Autodesk Inventor part; units mm, degrees
ref_plane "YZ Plane" through (0, 0, 0) normal (1, 0, 0) x (0, 1, 0)
ref_plane "XZ Plane" through (0, 0, 0) normal (0, 1, 0) x (-1, 0, 0)
ref_plane "XY Plane" through (0, 0, 0) normal (0, 0, 1) x (1, 0, 0)
sketch "Boceto1" plane through (0, 0, 0) normal (0, 1, 0) x (-1, 0, 0)
  circle A0 centre (0, 0) radius 11
  arc A1 (-35, 0) -> (27, 22.2711) centre (0, 0) ccw
  line L0 (-35, 0) -> (-35, 75)
  line L1 (-35, 75) -> (27, 75)
  line L2 (27, 75) -> (27, 22.2711)
  arc A2 (-11, 45) -> (11, 45) centre (0, 45) ccw
  arc A3 (11, 51) -> (-11, 51) centre (0, 51) ccw
  line L3 (11, 51) -> (11, 45)
  line L4 (-11, 45) -> (-11, 51)
  line L5 (15.5, 66.5) -> (15.5, 59.5) construction
  line L6 (13.95, 66.5) -> (13.95, 59.5)
  line L7 (17.05, 59.5) -> (17.05, 66.5)
  arc A4 (17.05, 66.5) -> (13.95, 66.5) centre (15.5, 66.5) ccw
  arc A5 (13.95, 59.5) -> (17.05, 59.5) centre (15.5, 59.5) ccw
  line L8 (0, 51) -> (0, 45)
  line L9 (0, 48) -> (2.6814, 48)
  line L10 (15.5, 29.5) -> (15.5, 36.5) construction
  line L11 (13.95, 29.5) -> (13.95, 36.5)
  line L12 (17.05, 36.5) -> (17.05, 29.5)
  arc A6 (13.95, 29.5) -> (17.05, 29.5) centre (15.5, 29.5) ccw
  arc A7 (17.05, 36.5) -> (13.95, 36.5) centre (15.5, 36.5) ccw
  line L13 (-15.5, 66.5) -> (-15.5, 59.5) construction
  line L14 (-13.95, 66.5) -> (-13.95, 59.5)
  line L15 (-17.05, 59.5) -> (-17.05, 66.5)
  arc A8 (-13.95, 66.5) -> (-17.05, 66.5) centre (-15.5, 66.5) ccw
  arc A9 (-17.05, 59.5) -> (-13.95, 59.5) centre (-15.5, 59.5) ccw
  line L16 (-13.95, 29.5) -> (-13.95, 36.5)
  line L17 (-15.5, 29.5) -> (-15.5, 36.5) construction
  line L18 (-17.05, 36.5) -> (-17.05, 29.5)
  arc A10 (-17.05, 29.5) -> (-13.95, 29.5) centre (-15.5, 29.5) ccw
  arc A11 (-13.95, 36.5) -> (-17.05, 36.5) centre (-15.5, 36.5) ccw
  point P0 (15.5, 63)
  point P1 (15.5, 33)
  point P2 (-15.5, 63)
  point P3 (-15.5, 33)
  dimension "d0" = 22
  dimension "d1" = 70
  dimension "d2" = 75
  dimension "d3" = 62
  dimension "d4" = 22
  dimension "d5" = 45
  dimension "d6" = 22
  dimension "d7" = 6
  dimension "d8" = 3.1
  dimension "d9" = 7
  dimension "d10" = 15.5
extrude "Extrusión1" add sketch "Boceto1" along normal blind 35
sketch "Boceto3" plane through (0, 0, 0) normal (0, -1, 0) x (1, 0, 0)
  line L0 (-21, 69) -> (21, 69)
  arc A0 (-21, 20) -> (21, 20) centre (0, 0) ccw
  line L1 (-27, 22.2711) -> (-27, 75)
  line L2 (-27, 75) -> (35, 75)
  line L3 (35, 75) -> (35, 0)
  line L4 (-21, 69) -> (-21, 20)
  line L5 (21, 69) -> (21, 20)
  dimension "d15" = 6
  dimension "d17" = 58
extrude "Extrusión2" cut sketch "Boceto3" against normal blind 28
sketch "Boceto4" plane through (0, 0, 0) normal (0, -1, 0) x (1, 0, 0)
  line L0 (-27, 75) -> (35, 75)
  line L1 (-27, 22.2711) -> (-27, 75)
  line L2 (27, 75) -> (-27, 75)
  line L3 (-27, 75) -> (-27, 69)
  line L4 (-27, 69) -> (27, 69)
  line L5 (27, 69) -> (27, 75)
  line L6 (-21, 69) -> (21, 69)
  line L7 (35, 75) -> (35, 0)
  line L8 (-20.5061, -20.5061) -> (-24.7487, -24.7487)
  arc A0 (-27, 22.2711) -> (35, 0) centre (0, 0) ccw
  line L9 (8.2115, 0) -> (-7.5561, 0)
  line L10 (-27, 22.2711) -> (-21, 22.2711)
  line L11 (-21, 20) -> (-21, 69)
  line L12 (-21, 22.2711) -> (-21, 20)
  arc A1 (-27, 22.2711) -> (-24.7487, -24.7487) centre (0, 0) ccw
  line L13 (20.5061, -20.5061) -> (24.7487, -24.7487)
  line L14 (21, 69) -> (21, 20)
  line L15 (21, 22.2711) -> (27, 22.2711)
  line L16 (21, 22.2711) -> (21, 20)
  arc A2 (20.5061, -20.5061) -> (21, 20) centre (0, 0) ccw
  arc A3 (24.7487, -24.7487) -> (27, 22.2711) centre (0, 0) ccw
  circle A4 centre (0, 0) radius 11
  line L17 (0, 2.7283) -> (0, -7.844)
  line L18 (7.5058, -28.0118) -> (9.0587, -33.8074)
  line L19 (-7.5058, -28.0118) -> (-9.0587, -33.8074)
  arc A5 (-7.5058, -28.0118) -> (7.5058, -28.0118) centre (0, 0) ccw
  arc A6 (-9.0587, -33.8074) -> (9.0587, -33.8074) centre (0, 0) ccw
  arc A7 (-21, 20) -> (-20.5061, -20.5061) centre (0, 0) ccw
  dimension "d20" = 0
  dimension "d21" = 8
  dimension "d22" = 45
  dimension "d24" = 35
  dimension "d25" = 45
extrude "Extrusión3" cut sketch "Boceto4" against normal blind 6 contours L0 L5 L4 L1 | L10 L11 A7 L8 A0 | A0 L13 A2 L14 L15 A3 | L19 A5 L18 A0
sketch "Boceto5" plane through (21, 28, 20) normal (-1, 0, 0) x (0, 0, 1)
  line L0 (49, -22) -> (49, 0)
  line L1 (2.2711, -22) -> (49, -22)
  circle A0 centre (10, -11.5) radius 3.1
  circle A1 centre (40, -11.5) radius 3.1
  line L2 (55, -22) -> (55, 7)
  line L3 (-20, -22) -> (-20, 7)
  point P0 (-20, -28)
  dimension "d30" = 6.2
  dimension "d31" = 30
  dimension "d32" = 15
  dimension "d33" = 10.5
  dimension "d34" = 10.5
  dimension "d50" = 30
extrude "Extrusión4" cut sketch "Boceto5" against normal up to next
sketch "Boceto6" plane through (21, 28, 20) normal (-1, 0, 0) x (0, 0, 1)
  circle A0 centre (40, -11.5) radius 3.1
  line L0 (37.0266, -16.65) -> (34.0533, -11.5)
  line L1 (34.0533, -11.5) -> (37.0266, -6.35)
  line L2 (37.0266, -6.35) -> (42.9734, -6.35)
  line L3 (42.9734, -6.35) -> (45.9467, -11.5)
  line L4 (45.9467, -11.5) -> (42.9734, -16.65)
  line L5 (42.9734, -16.65) -> (37.0266, -16.65)
  circle A1 centre (10, -11.5) radius 3.1
  line L6 (7.0266, -16.65) -> (4.0533, -11.5)
  line L7 (4.0533, -11.5) -> (7.0266, -6.35)
  line L8 (7.0266, -6.35) -> (12.9734, -6.35)
  line L9 (12.9734, -6.35) -> (15.9467, -11.5)
  line L10 (15.9467, -11.5) -> (12.9734, -16.65)
  line L11 (12.9734, -16.65) -> (7.0266, -16.65)
  line L12 (49, -28) -> (2.2711, -28)
  point P0 (-20, -28)
  dimension "d37" = 10.3
extrude "Extrusión5" cut sketch "Boceto6" against normal blind 4
fillet "Empalme1" radius 2 2 edges at (-27, 20.5, 75) (35, 17.5, 75)
fillet "Empalme2" radius 4 2 edges at (21, 17, 20) (-21, 17, 20)
sketch "Boceto8" plane through (0, 6, 0) normal (0, -1, 0) x (1, 0, 0)
  line L0 (-25, 75) -> (27, 75)
  line L1 (27, 75) -> (27, 69)
  line L2 (27, 75) -> (27, 69)
  line L3 (27, 69) -> (21, 69)
  line L4 (21, 22.2711) -> (27, 22.2711)
  line L5 (21, 69) -> (21, 22.2711)
  line L6 (21, 22.2711) -> (27, 22.2711)
  line L7 (24.7487, -24.7487) -> (20.5061, -20.5061)
  line L8 (24.7487, -24.7487) -> (20.5061, -20.5061)
  line L9 (20.5061, -20.5061) -> (24.7487, -24.7487)
  line L10 (7.5058, -28.0118) -> (9.0587, -33.8074)
  line L11 (7.5058, -28.0118) -> (9.0587, -33.8074)
  line L12 (-9.0587, -33.8074) -> (-7.5058, -28.0118)
  line L13 (-7.5058, -28.0118) -> (-9.0587, -33.8074)
  line L14 (-20.5061, -20.5061) -> (-24.7487, -24.7487)
  line L15 (-20.5061, -20.5061) -> (-24.7487, -24.7487)
  arc A0 (-27, 22.2711) -> (35, 0) centre (0, 0) ccw
  line L16 (-27, 22.2711) -> (-21, 22.2711)
  line L17 (-27, 22.2711) -> (-21, 22.2711)
  arc A1 (-27, 22.2711) -> (-24.7487, -24.7487) centre (0, 0) ccw
  arc A2 (-9.0587, -33.8074) -> (9.0587, -33.8074) centre (0, 0) ccw
  arc A3 (24.7487, -24.7487) -> (27, 22.2711) centre (0, 0) ccw
  arc A4 (20.5061, -20.5061) -> (21.9697, 18.9297) centre (0, 0) ccw
  arc A5 (7.5058, -28.0118) -> (20.5061, -20.5061) centre (0, 0) ccw
  arc A6 (-20.5061, -20.5061) -> (-7.5058, -28.0118) centre (0, 0) ccw
  circle A7 centre (0, 0) radius 11
  circle A8 centre (0, -32) radius 2
  circle A9 centre (29.8743, 10.8734) radius 2
  circle A10 centre (-29.8743, 10.8734) radius 2
  line L18 (-27, 69) -> (-27, 75)
  line L19 (-27, 69) -> (-27, 73)
  line L20 (-27, 75) -> (-25, 75)
  line L21 (-27, 69) -> (-21, 69)
  line L22 (-21, 69) -> (-21, 22.2711)
  line L23 (-21, 21.5407) -> (-21, 69)
  line L24 (-27, 22.2711) -> (-21, 22.2711)
  circle A11 centre (0, 72) radius 2
  circle A12 centre (0, 72) radius 2.05
  circle A13 centre (29.8743, 10.8734) radius 2.05
  circle A14 centre (0, -32) radius 2.05
  circle A15 centre (-29.8743, 10.8734) radius 2.05
  dimension "d51" = 6
  dimension "d52" = 46.7289
  dimension "d62" = 4.1
sketch "Boceto10" plane through (0, 6, 0) normal (0, -1, 0) x (1, 0, 0)
  circle A0 centre (0, 72) radius 2.05
  line L0 (6.7845, 0) -> (-6.2714, 0)
  circle A1 centre (0, 0) radius 32
  circle A2 centre (30.0702, 10.9446) radius 2.05
  circle A3 centre (0, -32) radius 2.05
  circle A4 centre (-30.0702, 10.9446) radius 2.05
  circle A5 centre (0, 0) radius 11
  line L1 (0, 0) -> (-30.0702, 10.9446)
  line L2 (0, 0) -> (30.0702, 10.9446)
  line L3 (-25, 75) -> (27, 75)
  dimension "d63" = 64
  dimension "d64" = 20
  dimension "d65" = 20
  dimension "d66" = 4.1
  dimension "d69" = 3
extrude "Extrusión8" cut sketch "Boceto10" against normal blind 5.8 contours A0 | A2 L2 A1 | A1 A2 | A3 A1 | A1 A3 | L2 A2 A1 | A4 A1 | A1 L1 A4 | A4 L1 A1
equation "\"d12\" = Altura"
equation "\"Altura\" = 35"
properties part number "Caja reductora - eje z" material "Plastico PETG"
Geometry check sheet. Reference: the model listing, model coordinates, mm. A direction names the side the tool comes from. Coordinates: 2 decimals unless noted, no trailing zeros. Write each loop counter-clockwise with the first axis right and the second up, starting at its lowest first coordinate (ties: lowest second). Pieces come first, ordered by that corner, then holes. Notation, with made-up numbers: M 29,-3.5 L 38,-3.5 A16 cw 38,8.5 Z; hole C 7.25,89.25 d4. An arc over 180 degrees is marked long. Use one line per item in the form item = value. Start each with the question number.
1) Section check D-D on z = -32. Enter the section's corners in (x, y), and give its area (3 significant figures).
2) Release check for a two-part mould opening along X. For faces 1 (the flat face through (-24, 3, 69)), 2 (the cylindrical face through (-12.71, 21.14, -32.61)), 3 (the flat face through (21, 14, 46)) record: pulls with the +X half, pulls with the -X half, needs draft (parallel to the pull), parting line crosses it, or undercut.
3) Go/stop test with flat-tipped pins: pin 1 Ø5.5 at (y, z) = (31, 33) entering from -X; pin 2 Ø5.5 at (x, z) = (0, -32) entering from -Y; pin 3 Ø2 at (x, y) = (17, 29.5) entering from -Z. Record where each tip stops, or that it passes through.
4) Section check C-C on z = 4.5. Enter the section's corners in (x, y), and give its area (3 significant figures).
5) Section check A-A on y = 31. Enter the section's corners in (x, z), and give its area (3 significant figures).
6) Set-up check for faces 4 (the flat face through (0, 17, 69)), 5 (the cylindrical face through (15.47, 31.45, 27.95)), 6 (the cylindrical face through (32.996, 2.958, 11.673)): record each of +Z, -Z, +X, -X, +Y, -Y from which the full face is reachable in a straight line by a thin tool's end or side.
7) Section check B-B on x = -4.5. Enter the section's corners in (y, z).
8) Thickness scan on probe 1 along Z at (x, y) = (0, 32); probe 2 along X at (y, z) = (31.75, 0); probe 3 along Z at (x, y) = (-3.5, 33.5). Record the ranges inside material, lowest first. Write a range as from..to.
Responses:
q1.outline = M -14.18,0 L -8.57,0 L -8.57,6 L -2.05,6 L -2.05,11.8 L 2.05,11.8 L 2.05,6 L 8.57,6 L 8.57,0 L 14.18,0 L 14.18,35 L -14.18,35 Z
q1.area = 866 mm2
q2.face_1 = needs draft
q2.face_2 = parting line crosses it
q2.face_3 = undercut
q3.pin_1 = -27
q3.pin_2 = 6
q3.pin_3 = -31.13
q4.outline = M -34.71,6 L -28.65,6 L -28.65,28 L -10.04,28 L -10.04,35 L -34.71,35 Z; M 10.04,28 L 28.65,28 L 28.65,6 L 34.71,6 L 34.71,0 L 35,0 L 35,35 L 10.04,35 Z
q4.area = 622 mm2
q5.outline = M -27,22.27 A35 ccw long 35,0 L 35,73 A2 ccw 33,75 L -25,75 A2 ccw -27,73 Z; hole M -17.05,29.5 A1.55 ccw -13.95,29.5 L -13.95,36.5 A1.55 ccw -17.05,36.5 Z; hole M -17.05,59.5 A1.55 ccw -13.95,59.5 L -13.95,66.5 A1.55 ccw -17.05,66.5 Z; hole C 0,0 d22; hole M -11,45 A11 ccw 11,45 L 11,51 A11 ccw -11,51 Z; hole M 13.95,29.5 A1.55 ccw 17.05,29.5 L 17.05,36.5 A1.55 ccw 13.95,36.5 Z; hole M 13.95,59.5 A1.55 ccw 17.05,59.5 L 17.05,66.5 A1.55 ccw 13.95,66.5 Z
q5.area = 5,690 mm2
q6.face_4 = -Y
q6.face_5 = +Y, -Y
q6.face_6 = -Z, -X, -Y
q7.outline = M 6,-34.71 L 35,-34.71 L 35,-10.04 L 28,-10.04 L 28,-28.65 L 6,-28.65 Z; M 6,69 L 28,69 L 28,61.04 L 35,61.04 L 35,75 L 6,75 Z; M 28,10.04 L 35,10.04 L 35,34.96 L 28,34.96 Z
q8.probe_1 = -35..-11, 11..34, 62..75
q8.probe_2 = -35..-11, 11..35
q8.probe_3 = -34.82..-10.43, 10.43..34.57, 61.43..75
